```python
from build123d import *

# Parameters (mm, degrees)
EXTRUDE_1_DEPTH     = 14
CUT_EXTRUDE_1_DEPTH = 44
SKETCH_3_W          = 6.2
SKETCH_3_H          = 6.2
CUT_EXTRUDE_2_DEPTH = 4
SKETCH_4_R          = 4
CUT_EXTRUDE_3_DEPTH = 5
SKETCH_5_R          = 2.6
CUT_EXTRUDE_4_DEPTH = 5
SKETCH_6_R          = 4
EXTRUDE_2_DEPTH     = 10
SKETCH_7_W          = 6.2
SKETCH_7_H          = 4
EXTRUDE_3_DEPTH     = 40
CUT_EXTRUDE_5_DEPTH = 50
SKETCH_9_W          = 20
SKETCH_9_H          = 25
EXTRUDE_4_DEPTH     = 44
CUT_EXTRUDE_6_DEPTH = 44
EXTRUDE_5_DEPTH     = 44
SKETCH_12_W         = 6.9
SKETCH_12_H         = 22.5
CUT_EXTRUDE_7_DEPTH = 50


with BuildPart() as part:
    # 草图1 → 凸台-拉伸1 (new body)
    with BuildSketch(Plane.XY):
        Polygon((-15, 22), (-15, -22), (15, -22), (15, 22), (0, 22), align=None)
    extrude(amount=EXTRUDE_1_DEPTH)

    # 草图2 → 切除-拉伸1 (cut)
    with BuildSketch(Plane(origin=(0, 22, 0), x_dir=(1, 0, 0), z_dir=(0, 1, 0))):
        Polygon((-15, 0), (-15, -14), (-10, -4), (-3.1, -4), (-3.1, 0), align=None)
        Polygon((3.1, -4), (10, -4), (15, -14), (15, 0), (3.1, 0), align=None)
    extrude(amount=-CUT_EXTRUDE_1_DEPTH, mode=Mode.SUBTRACT)

    # 草图3 → 切除-拉伸2 (cut)
    with BuildSketch(Plane(origin=(0, 0, 0), x_dir=(-1, 0, 0), z_dir=(0, 0, -1))):
        Rectangle(SKETCH_3_W, SKETCH_3_H)
    extrude(amount=-CUT_EXTRUDE_2_DEPTH, mode=Mode.SUBTRACT)

    # 草图4 → 切除-拉伸3 (cut)
    with BuildSketch(Plane.XY.offset(14)):
        Circle(SKETCH_4_R)
    extrude(amount=-CUT_EXTRUDE_3_DEPTH, mode=Mode.SUBTRACT)

    # 草图5 → 切除-拉伸4 (cut)
    with BuildSketch(Plane.XY.offset(9)):
        Circle(SKETCH_5_R)
    extrude(amount=-CUT_EXTRUDE_4_DEPTH, mode=Mode.SUBTRACT)

    # 草图6 → 凸台-拉伸2 (add)
    with BuildSketch(Plane.XY.offset(14)):
        Circle(SKETCH_6_R)
    extrude(amount=-EXTRUDE_2_DEPTH)

    # 草图7 → 凸台-拉伸3 (add)
    with BuildSketch(Plane(origin=(0, -22, 0), x_dir=(-1, 0, 0), z_dir=(0, -1, 0))):
        with Locations((0, -2)):
            Rectangle(SKETCH_7_W, SKETCH_7_H)
    extrude(amount=-EXTRUDE_3_DEPTH)

    # 草图8 → 切除-拉伸5 (cut)
    with BuildSketch(Plane.XZ.offset(22)):
        Polygon((-15, 14), (-10, 4), (-10, 14), align=None)
        Polygon((15, 14), (10, 14), (10, 4), align=None)
    extrude(amount=-CUT_EXTRUDE_5_DEPTH, mode=Mode.SUBTRACT)

    # 草图9 → 凸台-拉伸4 (add)
    with BuildSketch(Plane.XZ.offset(22)):
        with Locations((0, 16.5)):
            Rectangle(SKETCH_9_W, SKETCH_9_H)
    extrude(amount=-EXTRUDE_4_DEPTH)

    # 草图10 → 切除-拉伸6 (cut)
    with BuildSketch(Plane.XZ.offset(22)):
        with BuildLine():
            Line((-10, 29), (-10, 19))
            ThreePointArc((-10, 19), (-7.071067812, 26.071067812), (0, 29))
            Line((0, 29), (-10, 29))
        make_face()
    extrude(amount=-CUT_EXTRUDE_6_DEPTH, mode=Mode.SUBTRACT)

    # 草图11 → 凸台-拉伸5 (add)
    with BuildSketch(Plane.XZ.offset(22)):
        with BuildLine():
            Line((120, 0), (123.1, 0))
            Line((123.1, 0), (123.1, 4))
            Line((123.1, 4), (130, 4))
            Line((130, 4), (130, 19))
            ThreePointArc((130, 19), (127.071067812, 26.071067812), (120, 29))
            Line((120, 29), (110, 29))
            Line((110, 29), (10, 29))
            Line((10, 29), (10, 26.5))
            Line((10, 26.5), (110, 26.5))
            Line((110, 26.5), (110, 4))
            Line((110, 4), (116.9, 4))
            Line((116.9, 4), (116.9, 0))
            Line((116.9, 0), (120, 0))
        make_face()
    extrude(amount=-EXTRUDE_5_DEPTH)

    # 草图12 → 切除-拉伸7 (cut)
    with BuildSketch(Plane(origin=(0, 22, 0), x_dir=(1, 0, 0), z_dir=(0, 1, 0))):
        with Locations((6.55, -15.25)):
            Rectangle(SKETCH_12_W, SKETCH_12_H)
        with Locations((113.45, -15.25)):
            Rectangle(SKETCH_12_W, SKETCH_12_H)
    extrude(amount=-CUT_EXTRUDE_7_DEPTH, mode=Mode.SUBTRACT)


solid = part.part
```
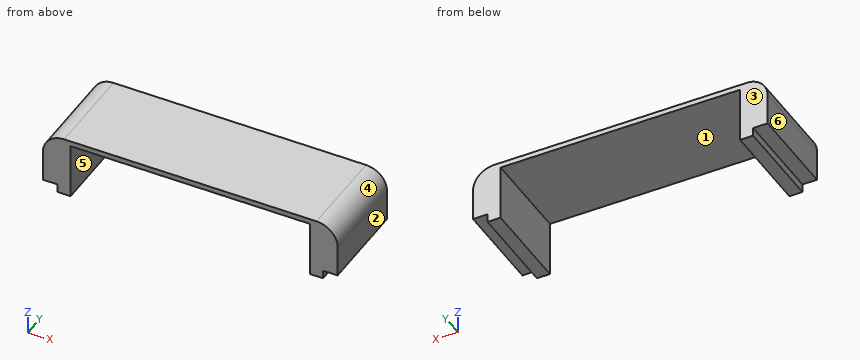
Can you work these out from the model? Positions are in its coordinate system, mm. Face numbers are marked on the shaded views. A direction names the side the tool comes from. Coordinates: 2 decimals unless noted, no trailing zeros. Loops run counter-clockwise (first coordinate to the right, second up) from the corner with the lowest first, then second, coordinate; pieces in that order, holes last. Notation, with made-up numbers: (32, 4) -> (55, 4) arc R22 ccw to (55, 15) -> close; hole circle Ø7 at (54, -1.75). An arc over 180 degrees is marked (long way). Put each result on its own line as item: value. Start each with the question number.
Q1. If I drill on line 1 (X direction, y = 3, z = 11.5); line 2 (X direction, y = 11.5, z = 2); line 3 (Z direction, x = 35.5, y = 19), over which ranges is the centre line in solid material (lowest first)? Write a range as [from, to].
Q2. I'm going to push flat-ended pins straight in: P1, Ø3, axis at x = 92.5, y = -8.5, coming from the -Z side; P2, Ø1.2, axis at y = 10, z = 2, coming from the -X side; P3, Ø1.2, axis at y = 1.5, z = 1, coming from the +X side. Where does each tip first touch, or does it pass through?
Q3. Thinking about a two-plate mould opening in X: for the marked faces 3, 4, 5 and 6, which applies, pulls with the +X half, pulls with the -X half, needs draft (parallel to the pull), parting line crosses it, or undercut?
Q4. I want a section at C-C (x = 96.5). Write out the boundary of the cut face in (y, z), plus the area to 3 significant figures.
Q5. For the marked faces 1 and 2, which set-ups out of +Z, -Z, +X, -X, +Y, -Y let a thin tool reach every point of the face, with its end or its side?
Q6. I want a section at B-B (y = -6.5). Write out the boundary of the cut face in (x, z).
Q7. I want a section at A-A (z = 7.5). Write out the boundary of the cut face in (x, y), plus the area to 3 significant figures.
Taken from the geometry:
1. line 1: x = [-10, 3.1], [116.9, 130]
1. line 2: x = [-3.1, 3.1], [116.9, 123.1]
1. line 3: z = [26.5, 29]
2. P1: stops at z = 26.5
2. P2: stops at x = -3.1
2. P3: stops at x = 123.1
3. face 3: needs draft
3. face 4: pulls with the +X half
3. face 5: undercut
3. face 6: pulls with the -X half
4. outline: (-22, 26.5) -> (22, 26.5) -> (22, 29) -> (-22, 29) -> close
4. area: 110 mm2
5. face 1: -Z, +Y, -Y
5. face 2: +Z, -Z, +X, +Y, -Y
6. outline: (-10, 4) -> (-3.1, 4) -> (-3.1, 0) -> (3.1, 0) -> (3.1, 26.5) -> (116.9, 26.5) -> (116.9, 0) -> (123.1, 0) -> (123.1, 4) -> (130, 4) -> (130, 19) arc R10 ccw to (120, 29) -> (0, 29) arc R10 ccw to (-10, 19) -> close
7. outline: (-10, -22) -> (3.1, -22) -> (3.1, 22) -> (-10, 22) -> close; (116.9, -22) -> (130, -22) -> (130, 22) -> (116.9, 22) -> close
7. area: 1,150 mm2
